from build123d import *

# Parameters (mm, degrees)
SKETCH1_R           = 3.26
BOSS_EXTRUDE1_DEPTH = 6.5
FILLET1_R           = 3.26
FILLET2_R           = 3.26


with BuildPart() as part:
    # Sketch1 → Boss-Extrude1 (new body)
    with BuildSketch(Plane(origin=(0, 0, 0), x_dir=(1, 0, 0), z_dir=(0, 1, 0))):
        with Locations(Location((0, 0, 0), (0, 0, 90))):
            Circle(SKETCH1_R)
    extrude(amount=BOSS_EXTRUDE1_DEPTH)

    # Fillet1
    fillet1_edges = [part.edges().sort_by_distance(p)[0] for p in [
        (0, 6.5, 3.26),
    ]]
    fillet(fillet1_edges, radius=FILLET1_R)

    # Fillet2
    # the kernel refuses this fillet: 3.26 mm, written as the material it takes off along each edge
    with BuildSketch(Plane(origin=(0, 0, 0), x_dir=(0, 0, -1), z_dir=(1, 0, 0))) as fillet2_piece_1:
        with BuildLine():
            CenterArc((6.135e-05, 3.26), FILLET2_R, 270, 89.648489945)
            Line((6.135e-05, 0), (6.135e-05, -0.0652))
            Line((6.135e-05, -0.0652), (3.26, -0.0652))
            Line((3.26, -0.0652), (3.3252, 0))
            Line((3.3252, 0), (3.325198773, 3.2396))
            Line((3.325198773, 3.2396), (3.26, 3.24))
        make_face()
    revolve(axis=Axis((0, 0, 0), (0, 1, 0)), mode=Mode.SUBTRACT)


solid = part.part
For this review, take the finished solid that the model builds, in its own axes (mm). Give positions to 0.01 mm unless a question says otherwise; leave off trailing zeros. Order: outer loops, then holes, each group sorted by start corner. A loop starts at its lowest first (then second) coordinate and runs counter-clockwise, first axis right, second up. Notation, with made-up numbers: M 80.25,53.5 L 99.25,53.5 A28 ccw 99.25,77.5 Z; hole C 3,38 d1. An arc over 180 degrees is marked long. Answer in a Markdown table with one row per item. Add a question column.
(1) Consider section B-B on y = 4.5. State the section outline as (x, z) points.
(2) Wall thickness on probe 1 along Z at (x, y) = (2.25, 2.75); probe 2 along Y at (x, z) = (-1.5, 0.25); probe 3 along Y at (x, z) = (-3, 0): over which ranges is each line inside the solid? List them lowest first. Write a range as [from, to].
(3) Consider section A-A on y = 3.5. State the section outline as (x, z) points.
(4) For pin 1 (2 mm diameter, centred on x = 0.5, y = 6, fed in from -Z); pin 2 (3 mm diameter, centred on x = -1.5, y = 4, fed in from +Z); pin 3 (1.5 mm diameter, centred on x = -2.5, z = 0.5, fed in from -Y), all flat-tipped, find the tip position at first contact; note any pin that passes through.
Evaluation:
| question | item | result |
|---|---|---|
| 1 | outline | C 0,0 d6.01 |
| 2 | probe 1 | z = [-2.3, 2.3] |
| 2 | probe 2 | y = [0.38, 6.12] |
| 2 | probe 3 | y = [1.98, 4.52] |
| 3 | outline | C 0,0 d6.5 |
| 4 | pin 1 | stops at z = -2.71 |
| 4 | pin 2 | stops at z = 3.25 |
| 4 | pin 3 | stops at y = 0.54 |
